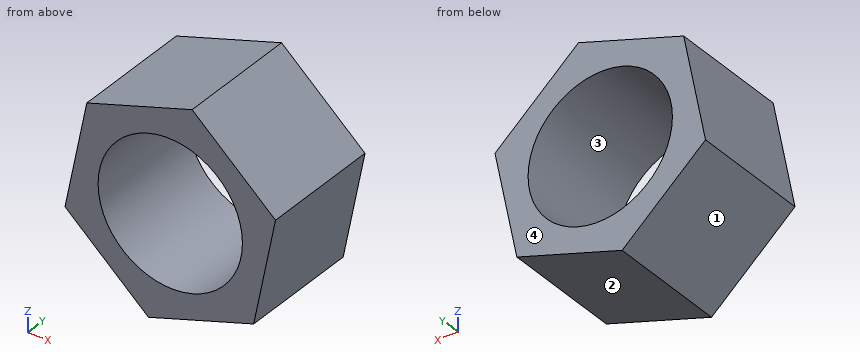
from build123d import *

# Parameters (mm, degrees)
F0_R     = 6
F1_DEPTH = 10


# Not quite as in the source:
# - the program builds the solid bodies; features that only make, move or delete a surface that nothing else refers to are left out


with BuildPart() as f1:
    # F0 (on Front) → F1 (new body)
    with BuildSketch(Plane.XZ):
        Polygon((-16.8017068945, -5.2552340917), (-8.0502918376, -2.2978589318), (-6.2357463262, 6.7597764064), (-13.1726158716, 12.8600365847), (-21.9240309284, 9.9026614248), (-23.7385764399, 0.8450260866), align=None)
        with Locations((-14.987161383, 3.8024012465)):
            Circle(F0_R, mode=Mode.SUBTRACT)
    extrude(amount=F1_DEPTH)


solid = f1.part
Design review of the part built by this model. Coordinates are the model's own, in mm. Face numbers are marked on the shaded views. Give positions to 0.01 mm unless a question says otherwise; leave off trailing zeros. Order: outer loops, then holes, each group sorted by start corner. A loop starts at its lowest first (then second) coordinate and runs counter-clockwise, first axis right, second up.
1. Mouldability with a two-part tool opening along X and no side actions: class the marked faces 1, 2, 3 and 4 as +X half, -X half, draft (parallel to the pull), parting line (faces both ways), or undercut.
Solution:
face 1: -X half
face 2: +X half
face 3: undercut
face 4: draft
2. Add section D-D, the plane x = -7.75. State the section outline as (y, z) points.
Solution:
outline: (-10, -0.8) - (0, -0.8) - (0, 8.09) - (-10, 8.09) - close
3. Add section C-C, the plane y = -7.5. State the section outline as (x, z) points.
Solution:
outline: (-23.74, 0.85) - (-16.8, -5.26) - (-8.05, -2.3) - (-6.24, 6.76) - (-13.17, 12.86) - (-21.92, 9.9) - close; hole circle Ø12 at (-14.99, 3.8)
4. Add section B-B, the plane x = -14.25. State the section outline as (y, z) points.
Solution:
outline: (-10, -4.39) - (0, -4.39) - (0, -2.15) - (-10, -2.15) - close; (-10, 9.76) - (0, 9.76) - (0, 12.5) - (-10, 12.5) - close
5. Add section A-A, the plane z = -1.25. State the section outline as (x, y) points, then the cut area to 3 significant figures.
Solution:
outline: (-21.36, -10) - (-18.22, -10) - (-18.22, 0) - (-21.36, 0) - close; (-11.75, -10) - (-7.84, -10) - (-7.84, 0) - (-11.75, 0) - close
area: 70.4 mm2
6. To check wall thickness, follow L1, parallel to Z at x = -11.5, y = -9.5 (3 decimals); L2, parallel to X at y = -4.75, z = 7.5; L3, parallel to X at y = -7.5, z = 5.25. State the ranges of each line that lie inside material, in increasing order.
Solution:
L1: z = -3.464 to -1.08, 8.685 to 11.389
L2: x = -22.41 to -19.71, -10.26 to -7.08
L3: x = -22.86 to -20.81, -9.16 to -6.54
7. For pin 1 Ø2 at (x, y) = (-13.5, -6.5) entering from -Z; pin 2 Ø3 at (x, y) = (-21.5, -8.5) entering from +Z; pin 3 Ø5 at (y, z) = (-1, 4) entering from -X, all flat-tipped, find the tip position at first contact; note any pin that passes through.
Solution:
pin 1: stops at z = -4.48
pin 2: stops at z = 10.55
pin 3: stops at x = -23.61
